Can you work these out from the model? Positions are in its coordinate system, mm. A direction names the side the tool comes from. Give positions to 0.01 mm unless a question says otherwise; leave off trailing zeros. Order: outer loops, then holes, each group sorted by start corner. A loop starts at its lowest first (then second) coordinate and runs counter-clockwise, first axis right, second up. Notation, with made-up numbers: M 83.25,-31.5 L 103.25,-31.5 A31 cw 103.25,-3.5 Z; hole C -11,13.5 d7. An arc over 180 degrees is marked long. One line per question, with ' | ' between items. Start each with the question number.
1) For faces 4 (the flat face through (50, -26, 27.442)), 5 (the flat face through (-8, -17, 10.17)), 6 (the flat face through (50, -17.399, 22)), which set-ups out of +Z, -Z, +X, -X, +Y, -Y let a thin tool reach every point of the face, with its end or its side?
2) If we section it at B-B, the plane y = -25: Please give me the cut outline in (x, z).
3) If we section it at D-D, the plane z = 6.75: Please give me the cut outline in (x, y).
4) If we section it at A-A, the plane x = 8.5: Please give me the cut outline in (y, z), plus the area to 3 significant figures.
5) I'm going to push flat-ended pins straight in: pin 1 Ø10 at (y, z) = (-16, 5) entering from -X; pin 2 Ø8.5 at (x, z) = (55, 21.5) entering from +Y; pin 3 Ø5 at (x, z) = (-39, 5) entering from +Y; pin 4 Ø17.5 at (x, y) = (-3, -20.5) entering from +Z. Where does each tip first touch, or does it pass through?
6) Please list where these lines run through material, in increasing order: line 1 along X through (y, z) = (-30, 22); line 2 along Z through (x, y) = (20.5, -3); line 3 along Z through (x, y) = (42.5, -5.5). Write a range as [from, to].
7) Thinking about a two-plate mould opening in Y: for faces 1 (the flat face through (-43, -19.808, 5)), 2 (the flat face through (-33.85, -10, 5)), 3 (the cylindrical face through (7.958, -12.483, 5.156)), which applies, +Y half, -Y half, draft (parallel to the pull), parting line (faces both ways), or undercut?
8) If we section it at C-C, the plane y = -4.5: Please give me the cut outline in (x, z), plus the area to 3 significant figures.
```python
from build123d import *

# Parameters (mm, degrees)
F0_W     = 114.3
F0_H     = 10.170036
F1_DEPTH = 34.798
F2_W     = 17.233886
F2_H     = 19.807858
F3_DEPTH = 25.4
F4_R     = 6.99841
F5_DEPTH = 25.4
F6_W     = 26.374524
F6_H     = 34.798
F7_DEPTH = 17.272
F8_W     = 26.374524
F8_H     = 17.399
F9_DEPTH = 10.414


with BuildPart() as f1:
    # F0 (on Front) → F1 (new body)
    with BuildSketch(Plane.XZ):
        with Locations((6.0662, 5.085018)):
            Rectangle(F0_W, F0_H)
    extrude(amount=F1_DEPTH)

    # F2 (on face) → F3 (cut)
    with BuildSketch(Plane.XY.offset(10.170036)):
        with Locations((-42.466857, -9.903929)):
            Rectangle(F2_W, F2_H)
    extrude(amount=-F3_DEPTH, mode=Mode.SUBTRACT)

    # F4 (on face) → F5 (cut)
    with BuildSketch(Plane.XY.offset(10.170036)):
        with Locations((8.868933, -19.421801)):
            Circle(F4_R)
    extrude(amount=-F5_DEPTH, mode=Mode.SUBTRACT)

    # F6 (on face) → F7 (join)
    with BuildSketch(Plane.XY.offset(10.170036)):
        with Locations((50.028938, -17.399)):
            Rectangle(F6_W, F6_H)
    extrude(amount=F7_DEPTH)

    # F8 (on face) → F9 (cut)
    with BuildSketch(Plane.XY.offset(27.442036)):
        with Locations((50.028938, -8.6995)):
            Rectangle(F8_W, F8_H)
    extrude(amount=-F9_DEPTH, mode=Mode.SUBTRACT)


solid = f1.part
```
Results found:
1) face 4: +Z, +X, -X, +Y, -Y | face 5: +Z, -X, +Y, -Y | face 6: +Z, +X, -X, +Y
2) outline: M -51.08,0 L 4.64,0 L 4.64,10.17 L -51.08,10.17 Z; M 13.1,0 L 63.22,0 L 63.22,27.44 L 36.84,27.44 L 36.84,10.17 L 13.1,10.17 Z
3) outline: M -51.08,-34.8 L 63.22,-34.8 L 63.22,0 L -33.85,0 L -33.85,-19.81 L -51.08,-19.81 Z; hole C 8.87,-19.42 d14
4) outline: M -34.8,0 L -26.41,0 L -26.41,10.17 L -34.8,10.17 Z; M -12.43,0 L 0,0 L 0,10.17 L -12.43,10.17 Z | area: 212 mm²
5) pin 1: stops at x = -51.08 | pin 2: stops at y = -17.4 | pin 3: stops at y = -19.81 | pin 4: stops at z = 10.17
6) line 1: x = [36.84, 63.22] | line 2: z = [0, 10.17] | line 3: z = [0, 17.03]
7) face 1: +Y half | face 2: draft | face 3: undercut
8) outline: M -33.85,0 L 63.22,0 L 63.22,17.03 L 36.84,17.03 L 36.84,10.17 L -33.85,10.17 Z | area: 1,170 mm²
